from build123d import *

# Parameters (mm, degrees)
F1_DEPTH     = 9
F2_R         = 4.5
F3_DEPTH     = 25
F4_W         = 57
F4_H         = 30
F5_DEPTH     = 25
F6_SIZE      = 5
F7_T1_DEPTH  = 227
F7_T3_DEPTH  = 107.8584149398
F7_T5_DEPTH  = 27.8584149398
F7_T7_DEPTH  = 140
F7_T10_ANGLE = 90
F7_T12_ANGLE = 90
F7_T14_ANGLE = 90
F7_T16_ANGLE = 90


# Not quite as in the source:
# - a fillet or chamfer that OpenCascade refuses, or shapes differently, is made with other operations: its cross-section is extruded or revolved along the edge and cut away or added


with BuildPart() as f1:
    # F0 (on Front) → F1 (new body)
    with BuildSketch(Plane.XZ):
        with BuildLine():
            Line((113.7409908921, 84.5945477496), (-113.2590091079, 84.5945477496))
            ThreePointArc((-113.2590091079, 84.5945477496), (-138.0077464495, 74.3432850912), (-148.2590091079, 49.5945477496))
            Line((-148.2590091079, 49.5945477496), (-148.2590091079, -90.4054522504))
            ThreePointArc((-148.2590091079, -90.4054522504), (-138.0077464495, -115.1541895919), (-113.2590091079, -125.4054522504))
            Line((-113.2590091079, -125.4054522504), (113.7409908921, -125.4054522504))
            ThreePointArc((113.7409908921, -125.4054522504), (138.4897282336, -115.1541895919), (148.7409908921, -90.4054522504))
            Line((148.7409908921, -90.4054522504), (148.7409908921, 49.5945477496))
            ThreePointArc((148.7409908921, 49.5945477496), (138.4897282336, 74.3432850912), (113.7409908921, 84.5945477496))
        make_face()
    extrude(amount=F1_DEPTH)

    # F2 (on face) → F3 (join)
    with BuildSketch(Plane.XZ.offset(9)):
        with Locations((101.7409908921, 69.5945477496)):
            Circle(F2_R)
        with Locations((76.7409908921, 69.5945477496)):
            Circle(F2_R)
    extrude(amount=F3_DEPTH)

    # F4 (on face) → F5 (cut)
    with BuildSketch(Plane.XZ.offset(9)):
        with Locations((120.2409908921, -60.4054522504)):
            Rectangle(F4_W, F4_H)
    extrude(amount=-F5_DEPTH, mode=Mode.SUBTRACT)

    # F6
    f6_edges = [f1.edges().sort_by_distance(p)[0] for p in [
        (0.240991, -9, 84.594548),
    ]]
    chamfer(f6_edges, length=F6_SIZE)

    # F7: chamfer of 5 on 9 edges, made by hand

    # F7_s2 → F7_t1 (cut)
    with BuildSketch(Plane.YZ.offset(-113.2590091079)):
        with BuildLine():
            Line((-5.1414213562, 84.7359691059), (0.1414213562, 79.4531263934))
            Line((0.1414213562, 79.4531263934), (0.2414213562, 79.4531263934))
            ThreePointArc((0.2414213562, 79.4531263934), (0.1, 82.0238370715), (0.1, 84.5945477496))
            Line((0.1, 84.5945477496), (0, 84.6945477496))
            ThreePointArc((0, 84.6945477496), (-2.5707106781, 84.6945477496), (-5.1414213562, 84.8359691059))
            Line((-5.1414213562, 84.8359691059), (-5.1414213562, 84.7359691059))
        make_face()
        with BuildLine():
            Line((0.1414213562, -120.2640308941), (-5.1414213562, -125.5468736066))
            Line((-5.1414213562, -125.5468736066), (-5.1414213562, -125.6468736066))
            ThreePointArc((-5.1414213562, -125.6468736066), (-2.5707106781, -125.5054522504), (0, -125.5054522504))
            Line((0, -125.5054522504), (0.1, -125.4054522504))
            ThreePointArc((0.1, -125.4054522504), (0.1, -122.8347415723), (0.2414213562, -120.2640308941))
            Line((0.2414213562, -120.2640308941), (0.1414213562, -120.2640308941))
        make_face()
    extrude(amount=F7_T1_DEPTH, mode=Mode.SUBTRACT)

    # F7_s4 → F7_t3 (cut)
    with BuildSketch(Plane.XY.offset(-58.2638671902)):
        with BuildLine():
            Line((143.5995695358, 0.1414213562), (148.8824122483, -5.1414213562))
            Line((148.8824122483, -5.1414213562), (148.9824122483, -5.1414213562))
            ThreePointArc((148.9824122483, -5.1414213562), (148.8409908921, -2.5707106781), (148.8409908921, 0))
            Line((148.8409908921, 0), (148.7409908921, 0.1))
            ThreePointArc((148.7409908921, 0.1), (146.1702802139, 0.1), (143.5995695358, 0.2414213562))
            Line((143.5995695358, 0.2414213562), (143.5995695358, 0.1414213562))
        make_face()
    extrude(amount=F7_T3_DEPTH, mode=Mode.SUBTRACT)

    # F7_s6 → F7_t5 (cut)
    with BuildSketch(Plane.XY.offset(-90.4054522504)):
        with BuildLine():
            Line((143.5995695358, 0.1414213562), (148.8824122483, -5.1414213562))
            Line((148.8824122483, -5.1414213562), (148.9824122483, -5.1414213562))
            ThreePointArc((148.9824122483, -5.1414213562), (148.8409908921, -2.5707106781), (148.8409908921, 0))
            Line((148.8409908921, 0), (148.7409908921, 0.1))
            ThreePointArc((148.7409908921, 0.1), (146.1702802139, 0.1), (143.5995695358, 0.2414213562))
            Line((143.5995695358, 0.2414213562), (143.5995695358, 0.1414213562))
        make_face()
    extrude(amount=F7_T5_DEPTH, mode=Mode.SUBTRACT)

    # F7_s8 → F7_t7 (cut)
    with BuildSketch(Plane.XY.offset(-90.4054522504)):
        with BuildLine():
            Line((-143.1175877517, 0.1414213562), (-148.4004304642, -5.1414213562))
            Line((-148.4004304642, -5.1414213562), (-148.5004304642, -5.1414213562))
            ThreePointArc((-148.5004304642, -5.1414213562), (-148.3590091079, -2.5707106781), (-148.3590091079, 0))
            Line((-148.3590091079, 0), (-148.2590091079, 0.1))
            ThreePointArc((-148.2590091079, 0.1), (-145.6882984298, 0.1), (-143.1175877517, 0.2414213562))
            Line((-143.1175877517, 0.2414213562), (-143.1175877517, 0.1414213562))
        make_face()
    extrude(amount=F7_T7_DEPTH, mode=Mode.SUBTRACT)

    # F7_s9 → F7_t10 (revolve, cut)
    with BuildSketch(Plane.XY.offset(49.5945477496)):
        with BuildLine():
            Line((148.8824122483, -5.1414213562), (143.5995695358, 0.1414213562))
            Line((143.5995695358, 0.1414213562), (143.5995695358, 0.2414213562))
            ThreePointArc((143.5995695358, 0.2414213562), (146.1702802139, 0.1), (148.7409908921, 0.1))
            Line((148.7409908921, 0.1), (148.8409908921, 0))
            ThreePointArc((148.8409908921, 0), (148.8409908921, -2.5707106781), (148.9824122483, -5.1414213562))
            Line((148.9824122483, -5.1414213562), (148.8824122483, -5.1414213562))
        make_face()
    revolve(axis=Axis((113.7409908921, 0, 49.5945477496), (0, -1, 0)), revolution_arc=F7_T10_ANGLE, mode=Mode.SUBTRACT)

    # F7_s11 → F7_t12 (revolve, cut)
    with BuildSketch(Plane.YZ.offset(113.7409908921)):
        with BuildLine():
            Line((0.1414213562, -120.2640308941), (-5.1414213562, -125.5468736066))
            Line((-5.1414213562, -125.5468736066), (-5.1414213562, -125.6468736066))
            ThreePointArc((-5.1414213562, -125.6468736066), (-2.5707106781, -125.5054522504), (0, -125.5054522504))
            Line((0, -125.5054522504), (0.1, -125.4054522504))
            ThreePointArc((0.1, -125.4054522504), (0.1, -122.8347415723), (0.2414213562, -120.2640308941))
            Line((0.2414213562, -120.2640308941), (0.1414213562, -120.2640308941))
        make_face()
    revolve(axis=Axis((113.7409908921, 0, -90.4054522504), (0, -1, 0)), revolution_arc=F7_T12_ANGLE, mode=Mode.SUBTRACT)

    # F7_s13 → F7_t14 (revolve, cut)
    with BuildSketch(Plane.XY.offset(-90.4054522504)):
        with BuildLine():
            Line((-143.1175877517, 0.1414213562), (-148.4004304642, -5.1414213562))
            Line((-148.4004304642, -5.1414213562), (-148.5004304642, -5.1414213562))
            ThreePointArc((-148.5004304642, -5.1414213562), (-148.3590091079, -2.5707106781), (-148.3590091079, 0))
            Line((-148.3590091079, 0), (-148.2590091079, 0.1))
            ThreePointArc((-148.2590091079, 0.1), (-145.6882984298, 0.1), (-143.1175877517, 0.2414213562))
            Line((-143.1175877517, 0.2414213562), (-143.1175877517, 0.1414213562))
        make_face()
    revolve(axis=Axis((-113.2590091079, 0, -90.4054522504), (0, -1, 0)), revolution_arc=F7_T14_ANGLE, mode=Mode.SUBTRACT)

    # F7_s15 → F7_t16 (revolve, cut)
    with BuildSketch(Plane.YZ.offset(-113.2590091079)):
        with BuildLine():
            Line((0.1414213562, 79.4531263934), (-5.1414213562, 84.7359691059))
            Line((-5.1414213562, 84.7359691059), (-5.1414213562, 84.8359691059))
            ThreePointArc((-5.1414213562, 84.8359691059), (-2.5707106781, 84.6945477496), (0, 84.6945477496))
            Line((0, 84.6945477496), (0.1, 84.5945477496))
            ThreePointArc((0.1, 84.5945477496), (0.1, 82.0238370715), (0.2414213562, 79.4531263934))
            Line((0.2414213562, 79.4531263934), (0.1414213562, 79.4531263934))
        make_face()
    revolve(axis=Axis((-113.2590091079, 0, 49.5945477496), (0, -1, 0)), revolution_arc=F7_T16_ANGLE, mode=Mode.SUBTRACT)


solid = f1.part
Read the model definition and answer for the solid it produces. Units are mm, in the model's axes. A direction names the side the tool comes from. Round coordinates to 2 decimals unless told otherwise and drop trailing zeros. Order: outer loops, then holes, each group sorted by start corner. A loop starts at its lowest first (then second) coordinate and runs counter-clockwise, first axis right, second up.
1) The part is cut by section C-C on y = -26. Write down the section's boundary in (x, z).
2) The part is cut by section A-A on z = 41.5. Write down the section's boundary in (x, y).
3) Flat-ended cylindrical pins translate along their axes: pin 1 (2.5 mm diameter, centred on y = -4.5, z = -59, fed in from +X); pin 2 (3 mm diameter, centred on x = -71.5, z = 38, fed in from -Y); pin 3 (1.5 mm diameter, centred on x = 32.5, y = -9, fed in from -Z). Find the tip coordinate at first contact, or state that the pin passes through.
4) For faces 1 (the face through (120, -5, -45.405)), 2 (the face through (135.7, -8.28, 71.08)), determine the directions among +Z, -Z, +X, -X, +Y, -Y from which every point of the face is accessible in a straight line to the end or side of a thin tool.
5) The part is cut by section B-B on x = -48.5. Write down the section's boundary in (y, z), plus the area to 3 significant figures.
6) Straight lines are drawn through the part: L1, parallel to Y at x = 69, z = -12; L2, parallel to Z at x = 77, y = -18.5; L3, parallel to X at y = -7, z = -53. For each, find the intervals that lie inside material, in ascending order.
7) The mould has two halves that part along X. Classify faces 3 (the face through (104.16, -21.32, 73.39)), 4 (the face through (73.424, -21.325, 72.636)), 5 (the face through (-135.22, -8.28, -111.89)), 6 (the face through (102, -34, 70)): released by +X, released by -X, zero draft, split by the parting line, or undercut.
Resolved:
1. outline: circle Ø9 at (76.74, 69.59); circle Ø9 at (101.74, 69.59)
2. outline: (-147.76, -4.5) - (-143.26, -9) - (143.74, -9) - (148.24, -4.5) - (143.74, 0) - (-143.26, 0) - close
3. pin 1: stops at x = 91.74
3. pin 2: stops at y = -9
3. pin 3: stops at z = -121.16
4. face 1: +X, +Y, -Y
4. face 2: +Z, +X, -Y
5. outline: (-9, -120.41) - (-4.5, -124.91) - (0, -120.41) - (0, 79.59) - (-4.5, 84.09) - (-9, 79.59) - close
5. area: 1,840 mm2
6. L1: y = -9 to 0
6. L2: z = 65.1 to 74.09
6. L3: x = -145.26 to 91.74
7. face 3: undercut
7. face 4: undercut
7. face 5: released by -X
7. face 6: zero draft
